Build history of the part. All positions in model axes, mm. A direction names the side the tool comes from. Round coordinates to 2 decimals unless told otherwise and drop trailing zeros. Write each loop counter-clockwise with the first axis right and the second up, starting at its lowest first coordinate (ties: lowest second). Pieces come first, ordered by that corner, then holes.
from build123d import *

# Parameters (mm, degrees)
BOSS_EXTRUDE2_DEPTH  = 7.62
CUT_EXTRUDE1_DEPTH   = 0.508
SKETCH4_W            = 1.524
SKETCH4_H            = 3.556
CUT_EXTRUDE2_DEPTH   = 0.508
BOSS_EXTRUDE8_DEPTH  = 7.62
BOSS_EXTRUDE10_DEPTH = 7.62
FILLET2_R            = 1.27
CUT_EXTRUDE4_DEPTH   = 7.62
FILLET4_R            = 1.27


with BuildPart() as part:
    # Sketch2 → Boss-Extrude2 (new body)
    with BuildSketch(Plane.XY):
        with BuildLine():
            ThreePointArc((-3.81, 0), (0, -3.81), (3.81, 0))
            Line((3.81, 0), (3.81, 8.636))
            ThreePointArc((3.81, 8.636), (3.363630735, 9.713630735), (2.286, 10.16))
            Line((2.286, 10.16), (-2.286, 10.16))
            ThreePointArc((-2.286, 10.16), (-3.363630735, 9.713630735), (-3.81, 8.636))
            Line((-3.81, 8.636), (-3.81, 0))
        make_face()
        with BuildLine():
            Line((-0.762, 0), (1.016, 0))
            ThreePointArc((1.016, 0), (-0.359210245, -0.950380976), (-0.762, 0.672020833))
            Line((-0.762, 0.672020833), (-0.762, 0))
        make_face(mode=Mode.SUBTRACT)
    extrude(amount=BOSS_EXTRUDE2_DEPTH)

    # Sketch3 → Cut-Extrude1 (cut)
    with BuildSketch(Plane.XY.offset(7.62)):
        with BuildLine():
            Line((-0.762, 0), (1.016, 0))
            ThreePointArc((1.016, 0), (0.950380976, 0.359210245), (0.762, 0.672020833))
            Line((0.762, 0.672020833), (0.762, 3.556))
            Line((0.762, 3.556), (-0.762, 3.556))
            Line((-0.762, 3.556), (-0.762, 0))
        make_face()
    extrude(amount=-CUT_EXTRUDE1_DEPTH, mode=Mode.SUBTRACT)

    # Sketch4 → Cut-Extrude2 (cut)
    with BuildSketch(Plane(origin=(0, 0, 0), x_dir=(-1, 0, 0), z_dir=(0, 0, -1))):
        with Locations((0, 1.778)):
            Rectangle(SKETCH4_W, SKETCH4_H)
    extrude(amount=-CUT_EXTRUDE2_DEPTH, mode=Mode.SUBTRACT)

    # Sketch7 → Cut-Revolve1 (revolve, cut)
    with BuildSketch(Plane(origin=(0, 0, 0), x_dir=(1, 0, 0), z_dir=(0, 1, 0))):
        Polygon((0, 0), (0, -7.62), (1.524, -7.62), (1.016, -7.112), (1.016, -0.508), (1.524, 0), align=None)
    revolve(axis=Axis((0, 0, 0), (0, 0, 1)), mode=Mode.SUBTRACT)

    # Sketch10 → Boss-Extrude8 (add)
    with BuildSketch(Plane.XY.offset(7.62)):
        with BuildLine():
            Line((-3.81, 0), (-6.985, 0))
            ThreePointArc((-6.985, 0), (0, -6.985), (6.985, 0))
            Line((6.985, 0), (3.81, 0))
            ThreePointArc((3.81, 0), (0, -3.81), (-3.81, 0))
        make_face()
    extrude(amount=-BOSS_EXTRUDE8_DEPTH)

    # Sketch14 → Boss-Extrude10 (add)
    with BuildSketch(Plane.XY.offset(7.62)):
        with BuildLine():
            ThreePointArc((3.81, -5.85441073), (0, -6.985), (-3.81, -5.85441073))
            Line((-3.81, -5.85441073), (-3.81, -6.745362036))
            ThreePointArc((-3.81, -6.745362036), (0, -7.747), (3.81, -6.745362036))
            Line((3.81, -6.745362036), (3.81, -5.85441073))
        make_face()
    extrude(amount=-BOSS_EXTRUDE10_DEPTH)

    # Fillet2
    fillet2_edges = [part.edges().sort_by_distance(p)[0] for p in [
        (-6.985, 0, 3.81),
        (6.985, 0, 3.81),
    ]]
    fillet(fillet2_edges, radius=FILLET2_R)

    # Sketch16 → Cut-Extrude4 (cut)
    with BuildSketch(Plane.XY.offset(7.62)):
        with BuildLine():
            Line((-3.81, 0), (-2.286, 10.16))
            ThreePointArc((-2.286, 10.16), (-3.363630735, 9.713630735), (-3.81, 8.636))
            Line((-3.81, 8.636), (-3.81, 0))
        make_face()
        with BuildLine():
            Line((2.286, 10.16), (3.81, 0))
            Line((3.81, 0), (3.81, 8.636))
            ThreePointArc((3.81, 8.636), (3.363630735, 9.713630735), (2.286, 10.16))
        make_face()
    extrude(amount=-CUT_EXTRUDE4_DEPTH, mode=Mode.SUBTRACT)

    # Fillet4
    fillet4_edges = [part.edges().sort_by_distance(p)[0] for p in [
        (-3.81, -5.85441073, 3.81),
        (3.81, -5.85441073, 3.81),
        (-3.81, 0, 3.81),
        (-2.286, 10.16, 3.81),
        (2.286, 10.16, 3.81),
        (3.81, 0, 3.81),
    ]]
    fillet(fillet4_edges, radius=FILLET4_R)


solid = part.part
1) Slice it at C-C (y = 6.75). Write the cut outline in (x, z).
Results:
outline: (-2.8, 0) - (2.8, 0) - (2.8, 7.62) - (-2.8, 7.62) - close
2) Which spindle directions (+Z, -Z, +X, -X, +Y, -Y) get a long thin tool onto all of the face, cutting with end or side? Do faces 1 (the flat face through (0, 2, 7.112)), 2 (the flat face through (0, 2, 0.508)), 3 (the cylindrical face through (-0.056, -7.747, 3.863)). Say none if no direction does.
Results:
face 1: +Z
face 2: -Z
face 3: +Z, -Z, -Y
3) Slice it at D-D (x = -4.5). Write the cut outline in (y, z).
Results:
outline: (-5.34, 0) - (0.07, 0) - (0.07, 7.62) - (-5.34, 7.62) - close
4) Slice it at B-B (z = 6). Write the cut outline in (x, y) (3 decimals), plus the area to 3 significant figures.
Results:
outline: (-6.81, -1.552) arc R6.985 ccw to (-4.298, -5.506) arc R1.27 cw to (-3.81, -6.507) - (-3.81, -6.745) arc R7.747 ccw to (3.81, -6.745) - (3.81, -6.507) arc R1.27 cw to (4.298, -5.506) arc R6.985 ccw to (6.81, -1.552) arc R1.27 ccw to (5.572, 0) - (4.904, 0) arc R1.27 cw to (3.648, 1.082) - (2.448, 9.078) arc R1.27 ccw to (1.192, 10.16) - (-1.192, 10.16) arc R1.27 ccw to (-2.448, 9.078) - (-3.648, 1.082) arc R1.27 cw to (-4.904, 0) - (-5.572, 0) arc R1.27 ccw to start; hole circle Ø2.032 at (0, 0)
area: 141 mm2
5) Wall check: L1, parallel to Y at x = 0, z = 3.25; L2, parallel to X at y = 0.75, z = 0.75; L3, parallel to X at y = 6.25, z = 6. Give the ranges that are in metal, low to high.
Results:
L1: y = -7.75 to -1.02, 1.02 to 10.16
L2: x = -3.75 to -0.69, 0.69 to 3.75
L3: x = -2.87 to 2.87
6) Slice it at A-A (x = 0). Write the cut outline in (y, z), plus the area to 3 significant figures.
Results:
outline: (-7.75, 0) - (-1.52, 0) - (-1.02, 0.51) - (-1.02, 7.11) - (-1.52, 7.62) - (-7.75, 7.62) - close; (1.02, 0.51) - (3.56, 0.51) - (3.56, 0) - (10.16, 0) - (10.16, 7.62) - (3.56, 7.62) - (3.56, 7.11) - (1.02, 7.11) - close
area: 118 mm2
7) Pin check, flat tips, straight feed: pin 1 Ø2.5 at (x, y) = (0, 0) entering from +Z; pin 2 Ø0.6 at (y, z) = (2.5, 0.5) entering from -X; pin 3 Ø1.7 at (x, y) = (0, 1.5) entering from -Z; pin 4 Ø3 at (x, z) = (3.5, 5) entering from -Y. Stop position of each tip, or through.
Results:
pin 1: stops at z = 7.35
pin 2: stops at x = -3.48
pin 3: stops at z = 0
pin 4: stops at y = -7.48
8) Mould opens along Y. For faces 4 (the cylindrical face through (-5.91, -3.72, 3.86)), 5 (the conical face through (-0.042, -1.153, 7.25)), 6 (the cylindrical face through (2.01, 9.86, 3.86)) say: released by +Y, released by -Y, zero draft, split by the parting line, or undercut.
Results:
face 4: released by -Y
face 5: undercut
face 6: released by +Y
